Part print with two shaded views. Sizes in mm from the minimum x, y, z corner. A direction names the side the tool comes from. Give positions to 0.01 mm unless a question says otherwise; leave off trailing zeros. Order: outer loops, then holes, each group sorted by start corner. A loop starts at its lowest first (then second) coordinate and runs counter-clockwise, first axis right, second up. Notation, with made-up numbers: (78.25, 38) -> (90.25, 38) arc R21 cw to (90.25, 42) -> close; hole circle Ø2 at (-24, 15.25). An arc over 180 degrees is marked (long way). Answer as CSV lines item,"result".
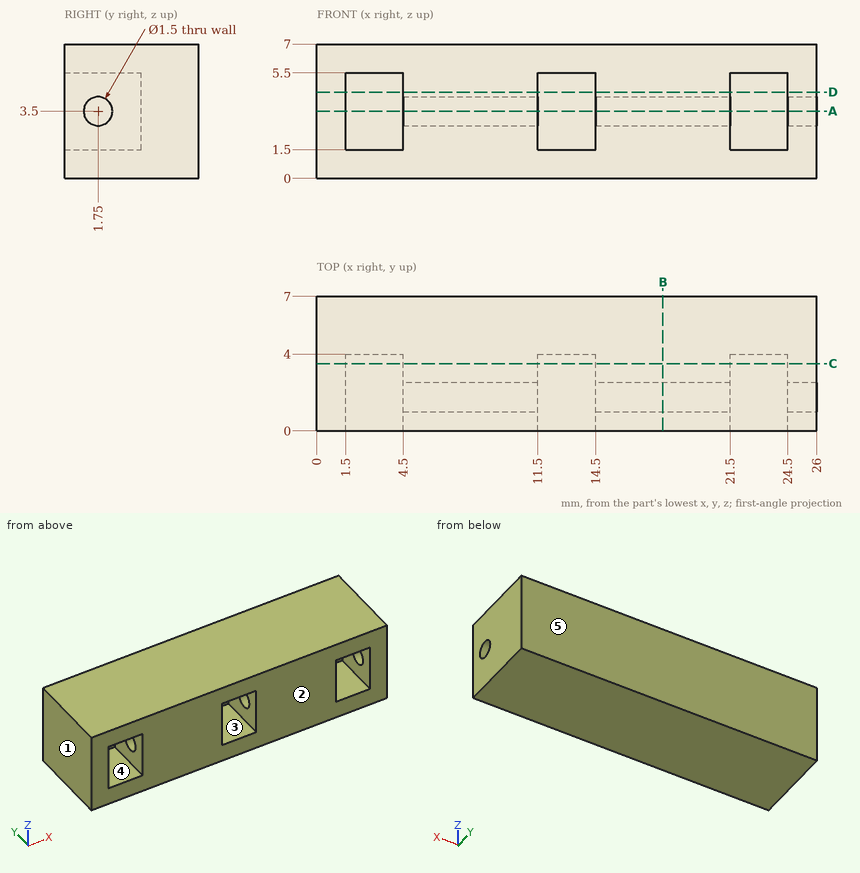
1) Which spindle directions (+Z, -Z, +X, -X, +Y, -Y) get a long thin tool onto all of the face, cutting with end or side? Do the marked faces 4 and 5. Say none if no direction does.
Data:
face 4,"-Y"
face 5,"+Z, -Z, +X, -X, +Y"
2) Pin check, flat tips, straight feed: P1, Ø1.5, axis at x = 22.5, z = 2.5, coming from the -Y side; P2, Ø0.9, axis at y = 1.75, z = 3.5, coming from the +X side. Stop position of each tip, or through.
Data:
P1,"stops at y = 4"
P2,"stops at x = 1.5"
3) Band-saw the part on D-D, the plane z = 4.5. Write the cut outline in (x, y).
Data:
outline,"(0, 0) -> (1.5, 0) -> (1.5, 4) -> (4.5, 4) -> (4.5, 0) -> (11.5, 0) -> (11.5, 4) -> (14.5, 4) -> (14.5, 0) -> (21.5, 0) -> (21.5, 4) -> (24.5, 4) -> (24.5, 0) -> (26, 0) -> (26, 7) -> (0, 7) -> close"
4) Band-saw the part on C-C, the plane y = 3.5. Write the cut outline in (x, z), then the cut area to 3 significant figures.
Data:
outline,"(0, 0) -> (26, 0) -> (26, 7) -> (0, 7) -> close; hole (1.5, 1.5) -> (4.5, 1.5) -> (4.5, 5.5) -> (1.5, 5.5) -> close; hole (11.5, 1.5) -> (14.5, 1.5) -> (14.5, 5.5) -> (11.5, 5.5) -> close; hole (21.5, 1.5) -> (24.5, 1.5) -> (24.5, 5.5) -> (21.5, 5.5) -> close"
area,"146 mm2"
5) Band-saw the part on A-A, the plane z = 3.5. Write the cut outline in (x, y).
Data:
outline,"(0, 0) -> (1.5, 0) -> (1.5, 4) -> (4.5, 4) -> (4.5, 2.5) -> (11.5, 2.5) -> (11.5, 4) -> (14.5, 4) -> (14.5, 2.5) -> (21.5, 2.5) -> (21.5, 4) -> (24.5, 4) -> (24.5, 2.5) -> (26, 2.5) -> (26, 7) -> (0, 7) -> close; (4.5, 0) -> (11.5, 0) -> (11.5, 1) -> (4.5, 1) -> close; (14.5, 0) -> (21.5, 0) -> (21.5, 1) -> (14.5, 1) -> close; (24.5, 0) -> (26, 0) -> (26, 1) -> (24.5, 1) -> close"
6) Pull direction X, two halves, no side cores. Call the marked faces 1, 2 and 3: pulls with the +X half, pulls with the -X half, needs draft (parallel to the pull), parting line crosses it, or undercut.
Data:
face 1,"pulls with the -X half"
face 2,"needs draft"
face 3,"undercut"
7) Wall check: line 1 along X through (y, z) = (1, 2); line 2 along Y through (x, z) = (23.5, 2); line 3 along Y through (x, z) = (17.5, 3.25). Give the ranges that are in metal, low to high. Write a range as [from, to].
Data:
line 1,"x = [0, 1.5], [4.5, 11.5], [14.5, 21.5], [24.5, 26]"
line 2,"y = [4, 7]"
line 3,"y = [0, 1.04], [2.46, 7]"
8) Band-saw the part on B-B, the plane x = 18. Write the cut outline in (y, z).
Data:
outline,"(0, 0) -> (7, 0) -> (7, 7) -> (0, 7) -> close; hole circle Ø1.5 at (1.75, 3.5)"
